```python
from build123d import *

# Parameters (mm, degrees)
SKETCH_1_W          = 32
SKETCH_1_H          = 42
SKETCH_1_W_2        = 2
SKETCH_1_H_2        = 38
EXTRUDE_1_DEPTH     = 3
SKETCH_2_R          = 1.5
CUT_EXTRUDE_1_DEPTH = 10


with BuildPart() as part:
    # 草图1 → 凸台-拉伸1 (new body)
    with BuildSketch(Plane.XY):
        Rectangle(SKETCH_1_W, SKETCH_1_H)
        with Locations((-17, 0)):
            Rectangle(SKETCH_1_W_2, SKETCH_1_H_2)
        with Locations((17, 0)):
            Rectangle(SKETCH_1_W_2, SKETCH_1_H_2)
    extrude(amount=EXTRUDE_1_DEPTH)

    # 草图2 → 切除-拉伸1 (cut)
    with BuildSketch(Plane.XY.offset(3)):
        with Locations((5.3, -7.6)):
            Circle(SKETCH_2_R)
        with Locations((5.3, 7.6)):
            Circle(SKETCH_2_R)
        with BuildLine():
            Line((-7.45, -10), (-7.45, 10))
            ThreePointArc((-7.45, 10), (-6.45, 11), (-5.45, 10))
            Line((-5.45, 10), (-5.45, -10))
            ThreePointArc((-5.45, -10), (-6.45, -11), (-7.45, -10))
        make_face()
    extrude(amount=-CUT_EXTRUDE_1_DEPTH, mode=Mode.SUBTRACT)


solid = part.part
```
Read the model definition and answer for the solid it produces. Units are mm, in the model's axes. A direction names the side the tool comes from. Coordinates: 2 decimals unless noted, no trailing zeros. Write each loop counter-clockwise with the first axis right and the second up, starting at its lowest first coordinate (ties: lowest second). Pieces come first, ordered by that corner, then holes. Notation, with made-up numbers: (18, 63) -> (38, 63) arc R18 cw to (38, 89) -> close; hole circle Ø3 at (76, 57). An arc over 180 degrees is marked (long way). Return JSON: item names as keys, results as strings.
1. A cutting plane is placed at C-C (y = -7.6). Determine the outline of the cut face in (x, z), and give its area (3 significant figures).
Found:
{"outline": "(-18, 0) -> (-7.45, 0) -> (-7.45, 3) -> (-18, 3) -> close; (-5.45, 0) -> (3.8, 0) -> (3.8, 3) -> (-5.45, 3) -> close; (6.8, 0) -> (18, 0) -> (18, 3) -> (6.8, 3) -> close", "area": "93.0 mm2"}
2. Find the intervals of material crossed by line 1 along Y through (x, z) = (5.3, 0.75); line 2 along X through (y, z) = (7, 2.65); line 3 along X through (y, z) = (3, 1.5), in increasing order. Write a range as from..to.
Found:
{"line 1": "-21..-9.1, -6.1..6.1, 9.1..21", "line 2": "-18..-7.45, -5.45..3.93, 6.67..18", "line 3": "-18..-7.45, -5.45..18"}
3. A tool of negligible diameter and unlimited length cuts with its end or side. For faces 4 (the face through (-17, -19, 1)), 5 (the face through (-17, 19, 1)), 6 (the face through (16, -20, 1)), 7 (the face through (-7.45, 0, 2)), 8 (the face through (-18, 0, 1)), from which of +Z, -Z, +X, -X, +Y, -Y can it reach the whole face along a straight path? Write none if from no direction.
Found:
{"face 4": "+Z, -Z, -X, -Y", "face 5": "+Z, -Z, -X, +Y", "face 6": "+Z, -Z, +X, -Y", "face 7": "+Z, -Z", "face 8": "+Z, -Z, -X, +Y, -Y"}
4. A cutting plane is placed at A-A (y = -3). Determine the outline of the cut face in (x, z).
Found:
{"outline": "(-18, 0) -> (-7.45, 0) -> (-7.45, 3) -> (-18, 3) -> close; (-5.45, 0) -> (18, 0) -> (18, 3) -> (-5.45, 3) -> close"}
5. A cutting plane is placed at D-D (x = 5.3). Determine the outline of the cut face in (y, z), and give its area (3 significant figures).
Found:
{"outline": "(-21, 0) -> (-9.1, 0) -> (-9.1, 3) -> (-21, 3) -> close; (-6.1, 0) -> (6.1, 0) -> (6.1, 3) -> (-6.1, 3) -> close; (9.1, 0) -> (21, 0) -> (21, 3) -> (9.1, 3) -> close", "area": "108 mm2"}
6. Determine the mould class of faces 1 (the face through (-6.4, -11, 1.5)), 2 (the face through (16, 20, 1)), 3 (the face through (17, 19, 1)) for opening direction X: pulls with the +X half, pulls with the -X half, needs draft (parallel to the pull), parting line crosses it, or undercut.
Found:
{"face 1": "undercut", "face 2": "pulls with the +X half", "face 3": "needs draft"}
7. Each of these flat-tipped pins is pushed along its axis until it touches: P1, Ø0.6, axis at x = 17.5, z = 2, coming from the +Y side; P2, Ø2.5, axis at x = 5.3, y = 7.6, coming from the -Z side; P3, Ø1.6, axis at x = -17, z = 1, coming from the -Y side. Where does it stop, or does it pass through?
Found:
{"P1": "y = 19", "P2": "through", "P3": "y = -19"}
8. A cutting plane is placed at B-B (x = -6.45). Determine the outline of the cut face in (y, z).
Found:
{"outline": "(-21, 0) -> (-11, 0) -> (-11, 3) -> (-21, 3) -> close; (11, 0) -> (21, 0) -> (21, 3) -> (11, 3) -> close"}
